For this review, take the finished solid that the model builds, in its own axes (mm). Face numbers are marked on the shaded views. A direction names the side the tool comes from. Coordinates: 2 decimals unless noted, no trailing zeros. Loops run counter-clockwise (first coordinate to the right, second up) from the corner with the lowest first, then second, coordinate; pieces in that order, holes last. Notation, with made-up numbers: M -25.5,-14 L -19.5,-14 A25 cw -19.5,5 Z; hole C 52,66.5 d7. An arc over 180 degrees is marked long. Answer as a JSON object with one key per item and string values. Group by question number.
Item 1: Wall thickness on L1, parallel to X at y = -58, z = 30; L2, parallel to Z at x = -11.5, y = 40; L3, parallel to Z at x = -3.5, y = 5: over which ranges is each line inside the solid? List them lowest first. Write a range as from..to.
Item 2: Add section D-D (y = -50). State the section outline as (x, z) points.
Item 3: Tool access review of the marked faces 4 and 5: name each direction out of +Z, -Z, +X, -X, +Y, -Y from which nothing blocks a thin tool from reaching the whole face with its end or side.
Item 4: Mouldability with a two-part tool opening along X and no side actions: class the marked faces 1, 2 and 3 as +X half, -X half, draft (parallel to the pull), parting line (faces both ways), or undercut.
Item 5: Insertion check: pin 1 (0.8 mm diameter, centred on x = 11.5, y = -47, fed in from -Z); pin 2 (0.8 mm diameter, centred on x = -11, y = -8.5, fed in from -Z); pin 3 (1.5 mm diameter, centred on x = 7.5, y = 24.5, fed in from -Z). Each pin has a flat end and moves straight along its axis. Give the tip position at first contact, or say it passes through.
Item 6: Add section C-C (x = -1.5). State the section outline as (y, z) points, then the cut area to 3 significant figures.
Item 7: Add section A-A (y = -7). State the section outline as (x, z) points.
Item 8: Add section B-B (z = 12.75). State the section outline as (x, y) points, then the cut area to 3 significant figures.
from build123d import *

# Parameters (mm, degrees)
F1_DEPTH     = 12.5
F2_SIZE      = 5
F3_T         = -2.5
F4_T1_DEPTH  = 2.5
F4_T3_DEPTH  = 2.5
F4_T5_DEPTH  = 2.5
F4_T7_DEPTH  = 2.5
F4_T9_DEPTH  = 13.1824295502
F4_T11_DEPTH = 13.1824295502
F4_T13_DEPTH = 12.5312469121
F4_T15_DEPTH = 12.5312469121
F4_T17_DEPTH = 10.2199869631
F4_T19_DEPTH = 10.2199869631
F4_T21_DEPTH = 13.4131081399
F4_T23_DEPTH = 13.4131081399
F4_T25_DEPTH = 12.0794727567
F4_T27_DEPTH = 12.0794727567
F4_T29_DEPTH = 13.6486136239
F4_T31_DEPTH = 13.6486136239
F6_DEPTH     = 12.5
F7_R         = 1


# Not quite as in the source:
# - a fillet or chamfer that OpenCascade refuses, or shapes differently, is made with other operations: its cross-section is extruded or revolved along the edge and cut away or added


with BuildPart() as f1:
    # F0 (on Right) → F1 (new body, symmetric)
    with BuildSketch(Plane.YZ):
        Polygon((64.5619183779, 36.750972271), (-66.8933242559, 36.750972271), (-66.8933242559, 24.738561362), (-61.0711984336, 19.1697143018), (-26.9197300076, 19.1697143018), (-18.7147669494, 24.7712358832), (14.4842416048, 24.7712358832), (28.7493690848, 9.385228157), (51.5191629529, 9.385228157), (64.5619183779, 21.1007967591), align=None)
    extrude(amount=F1_DEPTH, both=True)

    # F2
    f2_edges = [f1.edges().sort_by_distance(p)[0] for p in [
        (12.5, -1.165703, 36.750972),
        (-12.5, -1.165703, 36.750972),
    ]]
    chamfer(f2_edges, length=F2_SIZE)

    # F3
    f3_openings = [f1.faces().sort_by_distance(p)[0] for p in [
        (0, -66.893324, 30.350708),
        (0, -63.982261, 21.954138),
        (0, -43.995464, 19.169714),
        (0, -22.817248, 21.970475),
        (0, -2.115263, 24.771236),
        (0, 21.616805, 17.078232),
        (0, 40.134266, 9.385228),
        (0, 58.040541, 15.243012),
        (0, 64.561918, 28.50552),
    ]]
    offset(amount=F3_T, openings=f3_openings)

    # F4: fillet of radius 5 on 22 edges, made by hand

    # F4_s2 → F4_t1 (join)
    with BuildSketch(Plane.YZ.offset(-12.5)):
        with BuildLine():
            ThreePointArc((-19.9899366893, 23.9006785429), (-18.6460299918, 24.5486417325), (-17.1707695568, 24.7712358832))
            Line((-17.1707695568, 24.7712358832), (-18.7147669494, 24.7712358832))
            Line((-18.7147669494, 24.7712358832), (-19.9899366893, 23.9006785429))
        make_face()
    extrude(amount=F4_T1_DEPTH)

    # F4_s4 → F4_t3 (join)
    with BuildSketch(Plane.YZ.offset(10)):
        with BuildLine():
            ThreePointArc((-19.9899366893, 23.9006785429), (-18.6460299918, 24.5486417325), (-17.1707695568, 24.7712358832))
            Line((-17.1707695568, 24.7712358832), (-18.7147669494, 24.7712358832))
            Line((-18.7147669494, 24.7712358832), (-19.9899366893, 23.9006785429))
        make_face()
    extrude(amount=F4_T3_DEPTH)

    # F4_s6 → F4_t5 (join)
    with BuildSketch(Plane.YZ.offset(-12.5)):
        with BuildLine():
            ThreePointArc((12.3016199768, 24.7712358832), (14.3019608026, 24.3536628145), (15.9681862456, 23.1706905155))
            Line((15.9681862456, 23.1706905155), (14.4842416048, 24.7712358832))
            Line((14.4842416048, 24.7712358832), (12.3016199768, 24.7712358832))
        make_face()
    extrude(amount=F4_T5_DEPTH)

    # F4_s8 → F4_t7 (join)
    with BuildSketch(Plane.YZ.offset(10)):
        with BuildLine():
            ThreePointArc((12.3016199768, 24.7712358832), (14.3019608026, 24.3536628145), (15.9681862456, 23.1706905155))
            Line((15.9681862456, 23.1706905155), (14.4842416048, 24.7712358832))
            Line((14.4842416048, 24.7712358832), (12.3016199768, 24.7712358832))
        make_face()
    extrude(amount=F4_T7_DEPTH)

    # F4_s10 → F4_t9 (cut)
    with BuildSketch(Plane.YZ.offset(-17.8412147751)):
        with BuildLine():
            ThreePointArc((-66.8933242559, 26.8750472721), (-66.4911680254, 24.9104015861), (-65.3493911873, 23.2617937014))
            Line((-65.3493911873, 23.2617937014), (-66.8933242559, 24.738561362))
            Line((-66.8933242559, 24.738561362), (-66.8933242559, 26.8750472721))
        make_face()
    extrude(amount=F4_T9_DEPTH, mode=Mode.SUBTRACT)

    # F4_s12 → F4_t11 (cut)
    with BuildSketch(Plane.YZ.offset(4.6587852249)):
        with BuildLine():
            ThreePointArc((-66.8933242559, 26.8750472721), (-66.4911680254, 24.9104015861), (-65.3493911873, 23.2617937014))
            Line((-65.3493911873, 23.2617937014), (-66.8933242559, 24.738561362))
            Line((-66.8933242559, 24.738561362), (-66.8933242559, 26.8750472721))
        make_face()
    extrude(amount=F4_T11_DEPTH, mode=Mode.SUBTRACT)

    # F4_s14 → F4_t13 (cut)
    with BuildSketch(Plane.YZ.offset(-17.5156234561)):
        with BuildLine():
            ThreePointArc((-59.0649490512, 19.1697143018), (-60.9269012722, 19.5293335064), (-62.5210159826, 20.5564607312))
            Line((-62.5210159826, 20.5564607312), (-61.0711984336, 19.1697143018))
            Line((-61.0711984336, 19.1697143018), (-59.0649490512, 19.1697143018))
        make_face()
    extrude(amount=F4_T13_DEPTH, mode=Mode.SUBTRACT)

    # F4_s16 → F4_t15 (cut)
    with BuildSketch(Plane.YZ.offset(4.9843765439)):
        with BuildLine():
            ThreePointArc((-59.0649490512, 19.1697143018), (-60.9269012722, 19.5293335064), (-62.5210159826, 20.5564607312))
            Line((-62.5210159826, 20.5564607312), (-61.0711984336, 19.1697143018))
            Line((-61.0711984336, 19.1697143018), (-59.0649490512, 19.1697143018))
        make_face()
    extrude(amount=F4_T15_DEPTH, mode=Mode.SUBTRACT)

    # F4_s18 → F4_t17 (cut)
    with BuildSketch(Plane.YZ.offset(-16.3599934815)):
        with BuildLine():
            ThreePointArc((-25.6445602678, 20.0402716422), (-26.9884669653, 19.3923084525), (-28.4637274003, 19.1697143018))
            Line((-28.4637274003, 19.1697143018), (-26.9197300076, 19.1697143018))
            Line((-26.9197300076, 19.1697143018), (-25.6445602678, 20.0402716422))
        make_face()
    extrude(amount=F4_T17_DEPTH, mode=Mode.SUBTRACT)

    # F4_s20 → F4_t19 (cut)
    with BuildSketch(Plane.YZ.offset(6.1400065185)):
        with BuildLine():
            ThreePointArc((-25.6445602678, 20.0402716422), (-26.9884669653, 19.3923084525), (-28.4637274003, 19.1697143018))
            Line((-28.4637274003, 19.1697143018), (-26.9197300076, 19.1697143018))
            Line((-26.9197300076, 19.1697143018), (-25.6445602678, 20.0402716422))
        make_face()
    extrude(amount=F4_T19_DEPTH, mode=Mode.SUBTRACT)

    # F4_s22 → F4_t21 (cut)
    with BuildSketch(Plane.YZ.offset(-17.9565540699)):
        with BuildLine():
            ThreePointArc((30.9319907128, 9.385228157), (28.931649887, 9.8028012257), (27.2654244441, 10.9857735247))
            Line((27.2654244441, 10.9857735247), (28.7493690848, 9.385228157))
            Line((28.7493690848, 9.385228157), (30.9319907128, 9.385228157))
        make_face()
    extrude(amount=F4_T21_DEPTH, mode=Mode.SUBTRACT)

    # F4_s24 → F4_t23 (cut)
    with BuildSketch(Plane.YZ.offset(4.5434459301)):
        with BuildLine():
            ThreePointArc((30.9319907128, 9.385228157), (28.931649887, 9.8028012257), (27.2654244441, 10.9857735247))
            Line((27.2654244441, 10.9857735247), (28.7493690848, 9.385228157))
            Line((28.7493690848, 9.385228157), (30.9319907128, 9.385228157))
        make_face()
    extrude(amount=F4_T23_DEPTH, mode=Mode.SUBTRACT)

    # F4_s26 → F4_t25 (cut)
    with BuildSketch(Plane.YZ.offset(-17.2897363783)):
        with BuildLine():
            ThreePointArc((52.9444804464, 10.6655101473), (51.3923198194, 9.7162566403), (49.6032684016, 9.385228157))
            Line((49.6032684016, 9.385228157), (51.5191629529, 9.385228157))
            Line((51.5191629529, 9.385228157), (52.9444804464, 10.6655101473))
        make_face()
    extrude(amount=F4_T25_DEPTH, mode=Mode.SUBTRACT)

    # F4_s28 → F4_t27 (cut)
    with BuildSketch(Plane.YZ.offset(5.2102636217)):
        with BuildLine():
            ThreePointArc((52.9444804464, 10.6655101473), (51.3923198194, 9.7162566403), (49.6032684016, 9.385228157))
            Line((49.6032684016, 9.385228157), (51.5191629529, 9.385228157))
            Line((51.5191629529, 9.385228157), (52.9444804464, 10.6655101473))
        make_face()
    extrude(amount=F4_T27_DEPTH, mode=Mode.SUBTRACT)

    # F4_s30 → F4_t29 (cut)
    with BuildSketch(Plane.YZ.offset(4.425693188)):
        with BuildLine():
            ThreePointArc((64.5619183779, 23.3305194839), (64.128430188, 21.2941084527), (62.9031304227, 19.6108014742))
            Line((62.9031304227, 19.6108014742), (64.5619183779, 21.1007967591))
            Line((64.5619183779, 21.1007967591), (64.5619183779, 23.3305194839))
        make_face()
    extrude(amount=F4_T29_DEPTH, mode=Mode.SUBTRACT)

    # F4_s32 → F4_t31 (cut)
    with BuildSketch(Plane.YZ.offset(-18.074306812)):
        with BuildLine():
            ThreePointArc((64.5619183779, 23.3305194839), (64.128430188, 21.2941084527), (62.9031304227, 19.6108014742))
            Line((62.9031304227, 19.6108014742), (64.5619183779, 21.1007967591))
            Line((64.5619183779, 21.1007967591), (64.5619183779, 23.3305194839))
        make_face()
    extrude(amount=F4_T31_DEPTH, mode=Mode.SUBTRACT)

    # F5 (on Right) → F6 (cut, symmetric)
    with BuildSketch(Plane.YZ):
        Polygon((49.3934080005, 14.4370365888), (60.7276931405, 25.6640575826), (55.865034461, 25.6640575826), (44.530749321, 14.4370365888), align=None)
        Polygon((48.1250985598, 25.7630067087), (36.7908134197, 14.5359857149), (41.6534720992, 14.5359857149), (52.9877572393, 25.7630067087), align=None)
        Polygon((40.3851626585, 25.8619558348), (29.0508775185, 14.6349348409), (33.913536198, 14.6349348409), (45.247821338, 25.8619558348), align=None)
    extrude(amount=F6_DEPTH, both=True, mode=Mode.SUBTRACT)

    # F7
    f7_edges = [f1.edges().sort_by_distance(p)[0] for p in [
        (-11.25, 60.727693, 25.664058),
        (-11.25, 55.865034, 25.664058),
        (-11.25, 44.530749, 14.437037),
        (-11.25, 36.790813, 14.535986),
        (-11.25, 29.050878, 14.634935),
        (-11.25, 49.393408, 14.437037),
        (-11.25, 41.653472, 14.535986),
        (-11.25, 33.913536, 14.634935),
        (-11.25, 52.987757, 25.763007),
        (-11.25, 45.247821, 25.861956),
        (-11.25, 40.385163, 25.861956),
        (-11.25, 48.125099, 25.763007),
        (11.25, 60.727693, 25.664058),
        (11.25, 52.987757, 25.763007),
        (11.25, 45.247821, 25.861956),
        (11.25, 49.393408, 14.437037),
        (11.25, 41.653472, 14.535986),
        (11.25, 33.913536, 14.634935),
        (11.25, 40.385163, 25.861956),
        (11.25, 48.125099, 25.763007),
        (11.25, 55.865034, 25.664058),
        (11.25, 29.050878, 14.634935),
        (11.25, 36.790813, 14.535986),
        (11.25, 44.530749, 14.437037),
    ]]
    fillet(f7_edges, radius=F7_R)


solid = f1.part
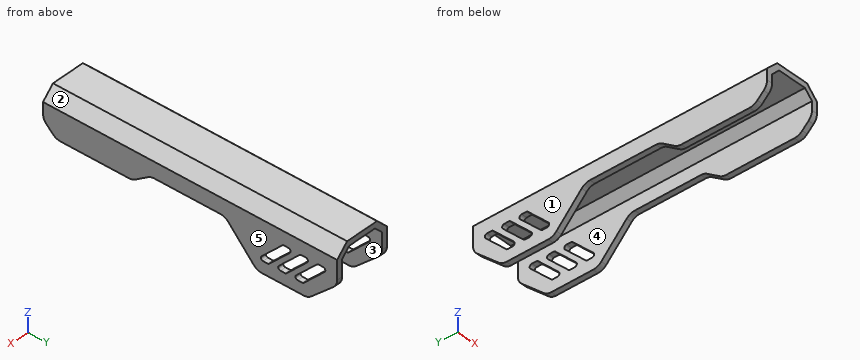
From the geometry:
{
 "1": {"L1": "x = -12.5..-10, 10..12.5", "L2": "z = 9.39..14.54, 17.71..20.66, 25.48..32.75", "L3": "z = 34.25..36.75"},
 "2": {"outline": "M -12.5,19.17 L -10,19.17 L -10,30.72 L -6.46,34.25 L 6.46,34.25 L 10,30.72 L 10,19.17 L 12.5,19.17 L 12.5,31.75 L 7.5,36.75 L -7.5,36.75 L -12.5,31.75 Z"},
 "3": {"face 4": "-Z, +Y, -Y", "face 5": "+Z, -Z, +X, +Y, -Y"},
 "4": {"face 1": "-X half", "face 2": "+X half", "face 3": "undercut"},
 "5": {"pin 1": "stops at z = 19.17", "pin 2": "stops at z = 24.77", "pin 3": "stops at z = 32.47"},
 "6": {"outline": "M -66.89,34.25 L 64.56,34.25 L 64.56,36.75 L -66.89,36.75 Z", "area": "329 mm²"},
 "7": {"outline": "M -12.5,24.77 L -10,24.77 L -10,30.72 L -6.46,34.25 L 6.46,34.25 L 10,30.72 L 10,24.77 L 12.5,24.77 L 12.5,31.75 L 7.5,36.75 L -7.5,36.75 L -12.5,31.75 Z"},
 "8": {"outline": "M -12.5,25.63 L -10,25.63 L -10,55.27 L -12.5,55.27 Z; M 10,25.63 L 12.5,25.63 L 12.5,55.27 L 10,55.27 Z", "area": "148 mm²"}
}
